```python
from build123d import *

# Parameters (mm, degrees)
SKETCH2_W           = 629.90984
SKETCH2_H           = 495.5921
SKETCH2_W_2         = 254
SKETCH2_H_2         = 3.175
SKETCH2_W_3         = 3.175
SKETCH2_H_3         = 76.2
BOSS_EXTRUDE1_DEPTH = 3.175
SKETCH4_W           = 28.585012188
SKETCH4_H           = 3.175
SKETCH4_W_2         = 62.54242
BOSS_EXTRUDE2_DEPTH = 3.175
SKETCH5_W           = 32.131
SKETCH5_H           = 106.20248
BOSS_EXTRUDE3_DEPTH = 3.175


with BuildPart() as part:
    # Sketch2 → Boss-Extrude1 (new body)
    with BuildSketch(Plane.XY):
        with Locations((313.68492, 246.52605)):
            Rectangle(SKETCH2_W, SKETCH2_H)
        with Locations((155.41371, 96.89592)):
            Rectangle(SKETCH2_W_2, SKETCH2_H_2, mode=Mode.SUBTRACT)
        with Locations((155.41371, 196.64934)):
            Rectangle(SKETCH2_W_2, SKETCH2_H_2, mode=Mode.SUBTRACT)
        with Locations((155.41371, 296.40276)):
            Rectangle(SKETCH2_W_2, SKETCH2_H_2, mode=Mode.SUBTRACT)
        with Locations((155.41371, 396.15618)):
            Rectangle(SKETCH2_W_2, SKETCH2_H_2, mode=Mode.SUBTRACT)
        with Locations((471.95613, 96.89592)):
            Rectangle(SKETCH2_W_2, SKETCH2_H_2, mode=Mode.SUBTRACT)
        with Locations((471.95613, 196.64934)):
            Rectangle(SKETCH2_W_2, SKETCH2_H_2, mode=Mode.SUBTRACT)
        with Locations((471.95613, 396.15618)):
            Rectangle(SKETCH2_W_2, SKETCH2_H_2, mode=Mode.SUBTRACT)
        with Locations((471.95613, 296.40276)):
            Rectangle(SKETCH2_W_2, SKETCH2_H_2, mode=Mode.SUBTRACT)
        with Locations((313.68492, 46.625498166)):
            Rectangle(SKETCH2_W_3, SKETCH2_H_3, mode=Mode.SUBTRACT)
        with Locations((313.68492, 146.77263)):
            Rectangle(SKETCH2_W_3, SKETCH2_H_3, mode=Mode.SUBTRACT)
        with Locations((313.68492, 246.52605)):
            Rectangle(SKETCH2_W_3, SKETCH2_H_3, mode=Mode.SUBTRACT)
        with Locations((313.68492, 346.27947)):
            Rectangle(SKETCH2_W_3, SKETCH2_H_3, mode=Mode.SUBTRACT)
        with Locations((313.68492, 446.03289)):
            Rectangle(SKETCH2_W_3, SKETCH2_H_3, mode=Mode.SUBTRACT)
    extrude(amount=BOSS_EXTRUDE1_DEPTH)

    # Sketch4 → Boss-Extrude2 (add, through all)
    with BuildSketch(Plane.XY.offset(3.175)):
        with Locations((13.022506094, -2.8575)):
            Rectangle(SKETCH4_W, SKETCH4_H)
        with Locations((614.347333906, -2.8575)):
            Rectangle(SKETCH4_W, SKETCH4_H)
        with Locations((313.68492, -2.8575)):
            Rectangle(SKETCH4_W_2, SKETCH4_H)
    extrude(amount=-BOSS_EXTRUDE2_DEPTH)

    # Sketch5 → Boss-Extrude3 (add, through all)
    with BuildSketch(Plane.XY.offset(3.175)):
        Polygon((158.03372, -20.246485543), (158.03372, -36.576), (-1.27, -36.576), (-1.27, -7.62), (-1.27, -4.445), (628.63984, -4.445), (628.63984, -7.62), (628.63984, -36.576), (469.33612, -36.576), (469.33612, -20.246485543), align=None)
        with Locations((644.70534, 438.04586)):
            Rectangle(SKETCH5_W, SKETCH5_H)
        with Locations((-17.3355, 438.04586)):
            Rectangle(SKETCH5_W, SKETCH5_H)
    extrude(amount=-BOSS_EXTRUDE3_DEPTH)


solid = part.part
```
The listing builds one solid part. Answer for the finished solid, in the listing's coordinates (mm). Give positions to 0.01 mm unless a question says otherwise; leave off trailing zeros. Order: outer loops, then holes, each group sorted by start corner. A loop starts at its lowest first (then second) coordinate and runs counter-clockwise, first axis right, second up.
1) Find section B-B on y = 266.5. Write down the section's boundary in (x, z) (3 decimals).
Reported:
outline: (-1.27, 0) - (312.097, 0) - (312.097, 3.175) - (-1.27, 3.175) - close; (315.272, 0) - (628.64, 0) - (628.64, 3.175) - (315.272, 3.175) - close
2) Find section D-D on z = 2.2. Give the number of separate pieces and of enclosed holes in the cut face, then the cut area to 3 significant figures.
Reported:
separate pieces: 1
enclosed holes: 15
area: 327,000 mm2
3) Given P1, Ø1.6, axis at y = 250, z = 2.5, coming from the +X side; P2, Ø1, axis at x = 647, z = 1.5, coming from the +Y side; P3, Ø1, axis at y = -3.5, z = 1, coming from the -X side, each flat-ended and moving along its own axis, determine where each tip first touches the part or whether it passes through.
Reported:
P1: stops at x = 628.64
P2: stops at y = 491.15
P3: stops at x = -1.27
4) Consider line 1 along Y through (x, z) = (50, 0.75) (3 decimals); line 2 along Y through (x, z) = (440.5, 0.4) (3 decimals); line 3 along X through (y, z) = (84, 0.2). Determine where each line is inside the solid, lowest interval first.
Reported:
line 1: y = -36.576 to -4.445, -1.27 to 95.308, 98.483 to 195.062, 198.237 to 294.815, 297.99 to 394.569, 397.744 to 494.322
line 2: y = -20.246 to -4.445, -1.27 to 95.308, 98.483 to 195.062, 198.237 to 294.815, 297.99 to 394.569, 397.744 to 494.322
line 3: x = -1.27 to 312.1, 315.27 to 628.64
5) Find section C-C on x = 443.5. Write down the section's boundary in (y, z) (3 decimals).
Reported:
outline: (-20.246, 0) - (-4.445, 0) - (-4.445, 3.175) - (-20.246, 3.175) - close; (-1.27, 0) - (95.308, 0) - (95.308, 3.175) - (-1.27, 3.175) - close; (98.483, 0) - (195.062, 0) - (195.062, 3.175) - (98.483, 3.175) - close; (198.237, 0) - (294.815, 0) - (294.815, 3.175) - (198.237, 3.175) - close; (297.99, 0) - (394.569, 0) - (394.569, 3.175) - (297.99, 3.175) - close; (397.744, 0) - (494.322, 0) - (494.322, 3.175) - (397.744, 3.175) - close
6) Find section A-A on x = 542. Write down the section's boundary in (y, z) (3 decimals).
Reported:
outline: (-36.576, 0) - (-4.445, 0) - (-4.445, 3.175) - (-36.576, 3.175) - close; (-1.27, 0) - (95.308, 0) - (95.308, 3.175) - (-1.27, 3.175) - close; (98.483, 0) - (195.062, 0) - (195.062, 3.175) - (98.483, 3.175) - close; (198.237, 0) - (294.815, 0) - (294.815, 3.175) - (198.237, 3.175) - close; (297.99, 0) - (394.569, 0) - (394.569, 3.175) - (297.99, 3.175) - close; (397.744, 0) - (494.322, 0) - (494.322, 3.175) - (397.744, 3.175) - close
